```python
from build123d import *

# Parameters (mm, degrees)
CYLINDER101_R             = 15
CYLINDER101_DEPTH         = 2.25
CYLINDER100_R             = 10.5
CYLINDER100_DEPTH         = 36
FUSION030_PLACEMENT_ANGLE = 90


with BuildPart() as ethernet003:
    # Cylinder101 → Cylinder101 (new body)
    with BuildSketch(Plane.XY.offset(13.5)):
        Circle(CYLINDER101_R)
    extrude(amount=CYLINDER101_DEPTH)


with BuildPart() as obj1:
    # Cylinder100 → Cylinder100 (new body)
    with BuildSketch(Plane.XY):
        Circle(CYLINDER100_R)
    extrude(amount=CYLINDER100_DEPTH)

    # Fusion030: union Ethernet003
    add(ethernet003.part)


with BuildPart() as obj1_1:
    # Fusion030 placement: moved
    add(obj1.part.moved(Location((34, 5, 124.5))).rotate(Axis((34, 5, 124.5), (0, -1, 0)), FUSION030_PLACEMENT_ANGLE))


solid = obj1_1.part
```
Model file for the job. Use its own axes, mm. A direction names the side the tool comes from. Round coordinates to 2 decimals unless told otherwise and drop trailing zeros. Order: outer loops, then holes, each group sorted by start corner. A loop starts at its lowest first (then second) coordinate and runs counter-clockwise, first axis right, second up. Notation, with made-up numbers: M 28,48 L 50,48 A16 cw 50,73 Z; hole C 16.5,35 d1. An arc over 180 degrees is marked long. Use CSV: the item, a comma, the result in double quotes.
Item 1: Probe probe 1 along X at (y, z) = (-3.5, 135); probe 2 along Y at (x, z) = (10, 128.5); probe 3 along Y at (x, z) = (24.5, 119). List the from-to ranges inside material, lowest first.
Worked answers:
probe 1,"18.25 to 20.5"
probe 2,"-4.71 to 14.71"
probe 3,"-3.94 to 13.94"
Item 2: Saw through at A-A (y = 5). List the corners of the cut face in (x, z).
Worked answers:
outline,"M -2,114 L 18.25,114 L 18.25,109.5 L 20.5,109.5 L 20.5,114 L 34,114 L 34,135 L 20.5,135 L 20.5,139.5 L 18.25,139.5 L 18.25,135 L -2,135 Z"
Item 3: Saw through at C-C (x = 15). List the corners of the cut face in (y, z).
Worked answers:
outline,"C 5,124.5 d21"
Item 4: Saw through at B-B (z = 124.5). List the corners of the cut face in (x, y).
Worked answers:
outline,"M -2,-5.5 L 18.25,-5.5 L 18.25,-10 L 20.5,-10 L 20.5,-5.5 L 34,-5.5 L 34,15.5 L 20.5,15.5 L 20.5,20 L 18.25,20 L 18.25,15.5 L -2,15.5 Z"
Item 5: Saw through at D-D (z = 113). List the corners of the cut face in (x, y), plus the area to 3 significant figures.
Worked answers:
outline,"M 18.25,-4.63 L 20.5,-4.63 L 20.5,14.63 L 18.25,14.63 Z"
area,"43.3 mm²"
Item 6: Pin check, flat tips, straight feed: pin 1 (1.5 mm diameter, centred on x = 6, z = 120.5, fed in from +Y); pin 2 (1 mm diameter, centred on x = 8, y = 0.5, fed in from +Z); pin 3 (6 mm diameter, centred on x = 21, y = 10.5, fed in from -Z). Stop position of each tip, or through.
Worked answers:
pin 1,"y = 14.98"
pin 2,"z = 134.21"
pin 3,"z = 109.72"
Item 7: Which spindle directions (+Z, -Z, +X, -X, +Y, -Y) get a long thin tool onto all of the face, cutting with end or side? Do faces 1 (the face through (27, 5, 114)), 2 (the face through (34, 5, 124)), 3 (the face through (8, 5, 114)). Say none if no direction does.
Worked answers:
face 1,"+X"
face 2,"+Z, -Z, +X, +Y, -Y"
face 3,"-X"
